Read the model definition and answer for the solid it produces. Units are mm, in the model's axes. A direction names the side the tool comes from. Give positions to 0.01 mm unless a question says otherwise; leave off trailing zeros. Order: outer loops, then holes, each group sorted by start corner. A loop starts at its lowest first (then second) coordinate and runs counter-clockwise, first axis right, second up.
```python
from build123d import *

# Parameters (mm, degrees)
SKETCH_1_R                        = 1.5
SM_BASE_FLANGE_2_DEPTH            = 1.5
SM_EDGE_FLANGE_2_STRIP_W          = 10
SM_EDGE_FLANGE_2_STRIP_H          = 1.5
SM_EDGE_FLANGE_2_STRIP_CUT_DEPTH  = 20
SM_EDGE_FLANGE_2_RELIEF_W         = 10.75
SM_EDGE_FLANGE_2_RELIEF_H         = 0.75
SM_EDGE_FLANGE_2_RELIEF_CUT_DEPTH = 1.5
SM_EDGE_FLANGE_2_DEPTH            = 20
SM_EDGE_FLANGE_2_PROFILE_R        = 1.5
SM_EDGE_FLANGE_2_FLAT_DEPTH       = 1.5
SM_EDGE_FLANGE_3_STRIP_W          = 10
SM_EDGE_FLANGE_3_STRIP_H          = 1.5
SM_EDGE_FLANGE_3_STRIP_CUT_DEPTH  = 20
SM_EDGE_FLANGE_3_RELIEF_W         = 10.75
SM_EDGE_FLANGE_3_RELIEF_H         = 0.75
SM_EDGE_FLANGE_3_RELIEF_CUT_DEPTH = 1.5
SM_EDGE_FLANGE_3_DEPTH            = 20
SM_EDGE_FLANGE_3_PROFILE_R        = 1.5
SM_EDGE_FLANGE_3_FLAT_DEPTH       = 1.5


# Sheet-metal steps are written as plain solids
with BuildPart() as part:
    # 草图1 → 基体-法兰2 (new body)
    with BuildSketch(Plane.XY):
        with BuildLine():
            Line((0, 34), (0, 22))
            Line((0, 22), (0, 10))
            Line((0, 10), (0, 7))
            Line((0, 7), (0, 2))
            ThreePointArc((0, 2), (0.585786438, 0.585786438), (2, 0))
            Line((2, 0), (38, 0))
            ThreePointArc((38, 0), (39.414213562, 0.585786438), (40, 2))
            Line((40, 2), (40, 61))
            ThreePointArc((40, 61), (39.414213562, 62.414213562), (38, 63))
            Line((38, 63), (34.32, 63))
            Line((34.32, 63), (4.32, 63))
            Line((4.32, 63), (2, 63))
            ThreePointArc((2, 63), (0.585786438, 62.414213562), (0, 61))
            Line((0, 61), (0, 41.32))
            Line((0, 41.32), (0, 37))
            Line((0, 37), (0, 34))
        make_face()
        with Locations((5.176021638, 36.143978362)):
            Circle(SKETCH_1_R, mode=Mode.SUBTRACT)
        with Locations((7.32, 41.32)):
            Circle(SKETCH_1_R, mode=Mode.SUBTRACT)
        with Locations((31.32, 41.32)):
            Circle(SKETCH_1_R, mode=Mode.SUBTRACT)
        with Locations((30.691436099, 35.076751631)):
            Circle(SKETCH_1_R, mode=Mode.SUBTRACT)
        with Locations((28.830973806, 29.08409589)):
            Circle(SKETCH_1_R, mode=Mode.SUBTRACT)
        with Locations((25.813288692, 23.582567072)):
            Circle(SKETCH_1_R, mode=Mode.SUBTRACT)
        with Locations((21.759505147, 18.792986533)):
            Circle(SKETCH_1_R, mode=Mode.SUBTRACT)
        with Locations((16.832334664, 14.907599318)):
            Circle(SKETCH_1_R, mode=Mode.SUBTRACT)
        with Locations((11.229544899, 12.082357801)):
            Circle(SKETCH_1_R, mode=Mode.SUBTRACT)
        with Locations((5.176021638, 5)):
            Circle(SKETCH_1_R, mode=Mode.SUBTRACT)
        with Locations((12.176021638, 5)):
            Circle(SKETCH_1_R, mode=Mode.SUBTRACT)
        with Locations((7.32, 55.66)):
            Circle(SKETCH_1_R, mode=Mode.SUBTRACT)
        with Locations((7.32, 48.66)):
            Circle(SKETCH_1_R, mode=Mode.SUBTRACT)
        with Locations((31.32, 55.66)):
            Circle(SKETCH_1_R, mode=Mode.SUBTRACT)
        with Locations((31.32, 48.66)):
            Circle(SKETCH_1_R, mode=Mode.SUBTRACT)
    extrude(amount=-SM_BASE_FLANGE_2_DEPTH)

    # 边线-法兰2 strip (across the edge) → 边线-法兰2 strip cut (cut)
    with BuildSketch(Plane(origin=(29.32, 63, 0), x_dir=(0, -1, 0), z_dir=(-1, 0, 0))):
        with Locations((-1.5, -0.75)):
            Rectangle(SM_EDGE_FLANGE_2_STRIP_W, SM_EDGE_FLANGE_2_STRIP_H)
    extrude(amount=SM_EDGE_FLANGE_2_STRIP_CUT_DEPTH, mode=Mode.SUBTRACT)

    # 边线-法兰2 relief (on the sheet) → 边线-法兰2 relief cut (cut)
    with BuildSketch(Plane(origin=(29.32, 59.5, 0), x_dir=(0, -1, 0), z_dir=(0, 0, 1))):
        with Locations((-4.625, 0.375)):
            Rectangle(SM_EDGE_FLANGE_2_RELIEF_W, SM_EDGE_FLANGE_2_RELIEF_H)
        with Locations((-4.625, -20.375)):
            Rectangle(SM_EDGE_FLANGE_2_RELIEF_W, SM_EDGE_FLANGE_2_RELIEF_H)
    extrude(amount=-SM_EDGE_FLANGE_2_RELIEF_CUT_DEPTH, mode=Mode.SUBTRACT)

    # 边线-法兰2 bend section (across the edge) → 边线-法兰2 (add)
    with BuildSketch(Plane(origin=(29.32, 63, 0), x_dir=(0, -1, 0), z_dir=(-1, 0, 0))):
        with BuildLine():
            Line((0, 2), (1.5, 2))
            ThreePointArc((1.5, 2), (2.085786438, 0.585786438), (3.5, 0))
            Line((3.5, 0), (3.5, -1.5))
            ThreePointArc((3.5, -1.5), (1.025126266, -0.474873734), (0, 2))
        make_face()
    extrude(amount=SM_EDGE_FLANGE_2_DEPTH)

    # 边线-法兰2 profile (on flange) → 边线-法兰2 flat (add)
    with BuildSketch(Plane(origin=(0, 63, 0), x_dir=(-1, 0, 0), z_dir=(0, 1, 0))):
        with BuildLine():
            Line((-29.32, 8), (-29.32, 2))
            Line((-29.32, 2), (-9.32, 2))
            Line((-9.32, 2), (-9.32, 8))
            ThreePointArc((-9.32, 8), (-9.905786438, 9.414213562), (-11.32, 10))
            Line((-11.32, 10), (-27.32, 10))
            ThreePointArc((-27.32, 10), (-28.734213562, 9.414213562), (-29.32, 8))
        make_face()
        with Locations((-24.32, 5)):
            Circle(SM_EDGE_FLANGE_2_PROFILE_R, mode=Mode.SUBTRACT)
        with Locations((-14.32, 5)):
            Circle(SM_EDGE_FLANGE_2_PROFILE_R, mode=Mode.SUBTRACT)
    extrude(amount=-SM_EDGE_FLANGE_2_FLAT_DEPTH)

    # 边线-法兰3 strip (across the edge) → 边线-法兰3 strip cut (cut)
    with BuildSketch(Plane.XZ.offset(-32)):
        with Locations((-1.5, -0.75)):
            Rectangle(SM_EDGE_FLANGE_3_STRIP_W, SM_EDGE_FLANGE_3_STRIP_H)
    extrude(amount=SM_EDGE_FLANGE_3_STRIP_CUT_DEPTH, mode=Mode.SUBTRACT)

    # 边线-法兰3 relief (on the sheet) → 边线-法兰3 relief cut (cut)
    with BuildSketch(Plane(origin=(3.5, 32, 0), x_dir=(1, 0, 0), z_dir=(0, 0, 1))):
        with Locations((-4.625, 0.375)):
            Rectangle(SM_EDGE_FLANGE_3_RELIEF_W, SM_EDGE_FLANGE_3_RELIEF_H)
        with Locations((-4.625, -20.375)):
            Rectangle(SM_EDGE_FLANGE_3_RELIEF_W, SM_EDGE_FLANGE_3_RELIEF_H)
    extrude(amount=-SM_EDGE_FLANGE_3_RELIEF_CUT_DEPTH, mode=Mode.SUBTRACT)

    # 边线-法兰3 bend section (across the edge) → 边线-法兰3 (add)
    with BuildSketch(Plane.XZ.offset(-32)):
        with BuildLine():
            Line((0, 2), (1.5, 2))
            ThreePointArc((1.5, 2), (2.085786438, 0.585786438), (3.5, 0))
            Line((3.5, 0), (3.5, -1.5))
            ThreePointArc((3.5, -1.5), (1.025126266, -0.474873734), (0, 2))
        make_face()
    extrude(amount=SM_EDGE_FLANGE_3_DEPTH)

    # 边线-法兰3 profile (on flange) → 边线-法兰3 flat (add)
    with BuildSketch(Plane(origin=(0, 0, 0), x_dir=(0, -1, 0), z_dir=(-1, 0, 0))):
        with BuildLine():
            Line((-32, 2), (-12, 2))
            Line((-12, 2), (-12, 8))
            ThreePointArc((-12, 8), (-12.585786438, 9.414213562), (-14, 10))
            Line((-14, 10), (-30, 10))
            ThreePointArc((-30, 10), (-31.414213562, 9.414213562), (-32, 8))
            Line((-32, 8), (-32, 2))
        make_face()
        with Locations((-17, 5)):
            Circle(SM_EDGE_FLANGE_3_PROFILE_R, mode=Mode.SUBTRACT)
        with Locations((-27, 5)):
            Circle(SM_EDGE_FLANGE_3_PROFILE_R, mode=Mode.SUBTRACT)
    extrude(amount=-SM_EDGE_FLANGE_3_FLAT_DEPTH)


solid = part.part
```
1) The part is cut by section D-D on z = 0.75. Determine the outline of the cut face in (x, y), and give its area (3 significant figures).
Final values:
outline: (0.23, 12) - (1.94, 12) - (1.94, 32) - (0.23, 32) - close; (9.32, 61.06) - (29.32, 61.06) - (29.32, 62.77) - (9.32, 62.77) - close
area: 68.3 mm2
2) For a pull along X with two mould halves and no side action, classify faces 3 (the face through (1.05, 22.14, -0.5)), 4 (the face through (19, 63, 6)), 5 (the face through (13.562, 4.425, -0.74)) as released by +X, released by -X, zero draft, split by the parting line, or undercut.
Final values:
face 3: released by -X
face 4: zero draft
face 5: undercut
3) Consider L1, parallel to Y at x = 7.32, z = -0.8; L2, parallel to Z at x = 3, y = 58.5; L3, parallel to Y at x = 19, z = 8.25. Determine where each line is inside the solid, lowest interval first.
Final values:
L1: y = 0 to 39.82, 42.82 to 47.16, 50.16 to 54.16, 57.16 to 63
L2: z = -1.5 to 0
L3: y = 61.5 to 63
4) The part is cut by section A-A on z = 5. Determine the outline of the cut face in (x, y), and give its area (3 significant figures).
Final values:
outline: (0, 12) - (1.5, 12) - (1.5, 15.5) - (0, 15.5) - close; (0, 18.5) - (1.5, 18.5) - (1.5, 25.5) - (0, 25.5) - close; (0, 28.5) - (1.5, 28.5) - (1.5, 32) - (0, 32) - close; (9.32, 61.5) - (12.82, 61.5) - (12.82, 63) - (9.32, 63) - close; (15.82, 61.5) - (22.82, 61.5) - (22.82, 63) - (15.82, 63) - close; (25.82, 61.5) - (29.32, 61.5) - (29.32, 63) - (25.82, 63) - close
area: 42.0 mm2
5) The part is cut by section C-C on x = 7.32. Determine the outline of the cut face in (y, z).
Final values:
outline: (0, -1.5) - (39.82, -1.5) - (39.82, 0) - (0, 0) - close; (42.82, -1.5) - (47.16, -1.5) - (47.16, 0) - (42.82, 0) - close; (50.16, -1.5) - (54.16, -1.5) - (54.16, 0) - (50.16, 0) - close; (57.16, -1.5) - (63, -1.5) - (63, 0) - (57.16, 0) - close
6) The part is cut by section B-B on y = 5. Determine the outline of the cut face in (x, z), and give its area (3 significant figures).
Final values:
outline: (0, -1.5) - (3.68, -1.5) - (3.68, 0) - (0, 0) - close; (6.68, -1.5) - (10.68, -1.5) - (10.68, 0) - (6.68, 0) - close; (13.68, -1.5) - (40, -1.5) - (40, 0) - (13.68, 0) - close
area: 51.0 mm2
7) A tool of negligible diameter and unlimited length cuts with its end or side. For faces 1 (the face through (1, 12, 2)), 2 (the face through (2.07, 22.14, 0.6)), from which of +Z, -Z, +X, -X, +Y, -Y can it reach the whole face along a straight path? Write none if from no direction.
Final values:
face 1: +Z, -Z, -X
face 2: +Z, +X, +Y, -Y
8) Given pin 1 (5 mm diameter, centred on x = 28.83, y = 29.08, fed in from +Z); pin 2 (1.3 mm diameter, centred on x = 2.5, z = 3.5, fed in from -Y); pin 3 (1.3 mm diameter, centred on y = 61.5, z = 2.5, fed in from -X); pin 4 (5 mm diameter, centred on x = 24.32, z = 5, fed in from -Y), each flat-ended and moving along its own axis, determine where each tip first touches the part or whether it passes through.
Final values:
pin 1: stops at z = 0
pin 2: passes through
pin 3: stops at x = 9.32
pin 4: stops at y = 61.5
